```python
from build123d import *

# Parameters (mm, degrees)
SKETCH1_W           = 72
SKETCH1_H           = 55
SKETCH1_W_2         = 90
SKETCH1_H_2         = 40
BOSS_EXTRUDE1_DEPTH = 6.5
FILLET1_R           = 20
FILLET2_R           = 30
SKETCH2_R           = 2.5
SKETCH2_R_2         = 2.59056518
SKETCH2_R_3         = 1.6
MOUNT_HOLES_DEPTH   = 132.02385279
SIDEWHEEL_CUT_REACH = 133.024
SKETCH3_W           = 10
SKETCH3_H           = 6.5
SKETCH4_W           = 20
SKETCH4_H           = 6.5
CROSSBAR_CUT_DEPTH  = 132.02385279


with BuildPart() as part:
    # Sketch1 → Boss-Extrude1 (new body)
    with BuildSketch(Plane.XY):
        with Locations((45, 67.5)):
            Rectangle(SKETCH1_W, SKETCH1_H)
        with Locations((45, 20)):
            Rectangle(SKETCH1_W_2, SKETCH1_H_2)
    extrude(amount=BOSS_EXTRUDE1_DEPTH)

    # Fillet1
    fillet1_edges = [part.edges().sort_by_distance(p)[0] for p in [
        (9, 95, 3.25),
        (81, 95, 3.25),
    ]]
    fillet(fillet1_edges, radius=FILLET1_R)

    # Fillet2
    fillet2_edges = [part.edges().sort_by_distance(p)[0] for p in [
        (90, 0, 3.25),
        (0, 0, 3.25),
    ]]
    fillet(fillet2_edges, radius=FILLET2_R)

    # Sketch2 → mount holes (cut, through all)
    with BuildSketch(Plane.XY.offset(6.5)):
        with Locations((25, 75)):
            Circle(SKETCH2_R)
        with Locations((65, 75)):
            Circle(SKETCH2_R)
        with Locations((45, 52.639320225)):
            Circle(SKETCH2_R_2)
        with Locations((62.960512242, 52.639320225)):
            Circle(SKETCH2_R_3)
        with Locations((45, 34.678807983)):
            Circle(SKETCH2_R_3)
        with Locations((27.039487758, 52.639320225)):
            Circle(SKETCH2_R_3)
    extrude(amount=-MOUNT_HOLES_DEPTH, mode=Mode.SUBTRACT)

    # Sketch3 → sidewheel cut (cut, up to next)
    with BuildSketch(Plane.XY.offset(6.5), mode=Mode.PRIVATE) as sidewheel_cut_sk1:
        with Locations((24, 43.25)):
            Rectangle(SKETCH3_W, SKETCH3_H)
    sidewheel_cut_tool1 = extrude(sidewheel_cut_sk1.sketch, amount=-SIDEWHEEL_CUT_REACH, mode=Mode.PRIVATE) & part.part
    # Sketch3 → sidewheel cut (cut, up to next)
    with BuildSketch(Plane.XY.offset(6.5), mode=Mode.PRIVATE) as sidewheel_cut_sk2:
        with Locations((66, 43.25)):
            Rectangle(SKETCH3_W, SKETCH3_H)
    sidewheel_cut_tool2 = extrude(sidewheel_cut_sk2.sketch, amount=-SIDEWHEEL_CUT_REACH, mode=Mode.PRIVATE) & part.part
    add(sidewheel_cut_tool1.solids().sort_by_distance((24, 43.25, 6.5))[0], mode=Mode.SUBTRACT)
    add(sidewheel_cut_tool2.solids().sort_by_distance((66, 43.25, 6.5))[0], mode=Mode.SUBTRACT)

    # Sketch4 → crossbar cut (cut, through all)
    with BuildSketch(Plane.XY.offset(6.5)):
        with Locations((45, 22.75)):
            Rectangle(SKETCH4_W, SKETCH4_H)
        with Locations((45, 9.75)):
            Rectangle(SKETCH4_W, SKETCH4_H)
    extrude(amount=-CROSSBAR_CUT_DEPTH, mode=Mode.SUBTRACT)


solid = part.part
```
Geometry: final body of the model. Coordinates: model frame, mm. A direction names the side the tool comes from. Round coordinates to 2 decimals unless told otherwise and drop trailing zeros. Order: outer loops, then holes, each group sorted by start corner. A loop starts at its lowest first (then second) coordinate and runs counter-clockwise, first axis right, second up. Notation, with made-up numbers: (26.25, 1.5) - (75.25, 1.5) arc R18 cw to (75.25, 20.5) - close; hole circle Ø9 at (16, 78). An arc over 180 degrees is marked (long way). Use CSV: the item, a comma, the result in double quotes. Start each with the question number.
Q1. Section query A-A (y = 44). Return loops of the section in (x, z).
Q2. First-contact query: pin 1 (2 mm diameter, centred on x = 85.5, z = 3, fed in from +Y); pin 2 (3 mm diameter, centred on y = 63.5, z = 4, fed in from +X); pin 3 (2 mm diameter, centred on y = 43, z = 5, fed in from -X). Flat tips, straight axial feed; report the tip coordinate or a pass-through.
Q3. Section query C-C (y = 8). Return loops of the section in (x, z), and give its area (3 significant figures).
Q4. Mould query, pull axis X, two halves, no side actions, for faces 1 (the face through (4, 40, 3)), 2 (the face through (45.74, 33.26, 3.3)), 3 (the face through (0, 35, 3)). Classes: +X half, -X half, draft (parallel to the pull), parting line (faces both ways), or undercut.
Q5. Access query for faces 4 (the face through (35, 10, 3)), 5 (the face through (45, 95, 3)), 6 (the face through (9, 57, 3)). Directions: +Z, -Z, +X, -X, +Y, -Y. A direction counts if a zero-diameter tool reaches every point of the face in a straight line with its end or side. Return the directions, or none.
Q6. Section query B-B (x = 69.5). Return loops of the section in (y, z), and give its area (3 significant figures).
Q7. Material intervals for line 1 along X through (y, z) = (42.5, 5); line 2 along Y through (x, z) = (45, 3); line 3 along Y through (x, z) = (54, 2.5), sorted ascending. Write a range as from..to.
Q8. Section query D-D (z = 1.25). State how many separate pieces and enclosed holes the cut face has, and give its area (3 significant figures).
Result set:
1,outline,"(9, 0) - (19, 0) - (19, 6.5) - (9, 6.5) - close; (29, 0) - (61, 0) - (61, 6.5) - (29, 6.5) - close; (71, 0) - (81, 0) - (81, 6.5) - (71, 6.5) - close"
2,pin 1,"stops at y = 40"
2,pin 2,"stops at x = 81"
2,pin 3,"stops at x = 9"
3,outline,"(9.6, 0) - (35, 0) - (35, 6.5) - (9.6, 6.5) - close; (55, 0) - (80.4, 0) - (80.4, 6.5) - (55, 6.5) - close"
3,area,"330 mm2"
4,face 1,"draft"
4,face 2,"undercut"
4,face 3,"-X half"
5,face 4,"+Z, -Z"
5,face 5,"+Z, -Z, +X, -X, +Y"
5,face 6,"+Z, -Z, -X, +Y"
6,outline,"(1.54, 0) - (40, 0) - (40, 6.5) - (1.54, 6.5) - close; (46.5, 0) - (93.1, 0) - (93.1, 6.5) - (46.5, 6.5) - close"
6,area,"553 mm2"
7,line 1,"x = 9..19, 29..61, 71..81"
7,line 2,"y = 0..6.5, 13..19.5, 26..33.08, 36.28..50.05, 55.23..95"
7,line 3,"y = 0..6.5, 13..19.5, 26..95"
8,separate pieces,"1"
8,enclosed holes,"10"
8,area,"6,530 mm2"
